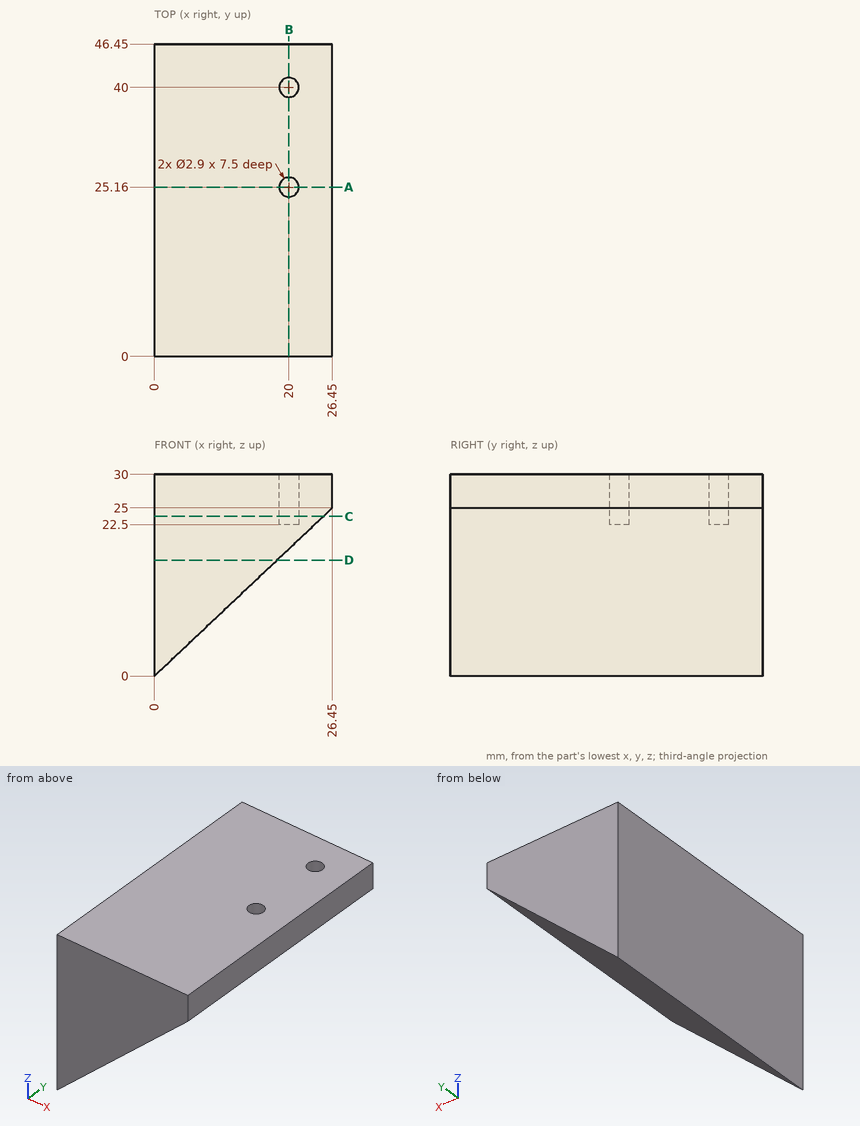
Answer from the drawing. Dimensions are ordinates in mm from the lowest x, y and z of the part. Round coordinates to 2 decimals unless told otherwise and drop trailing zeros. Write each loop counter-clockwise with the first axis right and the second up, starting at its lowest first coordinate (ties: lowest second). Pieces come first, ordered by that corner, then holes.
1. The part is cut by section B-B, the plane x = 20. Determine the outline of the cut face in (y, z).
2. Given pin 1 Ø12 at (y, z) = (15, 6.5) entering from +X (3 decimals); pin 2 Ø10 at (x, y) = (23, 11.5) entering from -Z; pin 3 Ø2.5 at (x, y) = (20, 25) entering from +Z, each flat-ended and moving along its own axis, determine where each tip first touches the part or whether it passes through.
3. The part is cut by section A-A, the plane y = 25.16. Determine the outline of the cut face in (x, z).
4. The part is cut by section D-D, the plane z = 17.25. Determine the outline of the cut face in (x, y), then the cut area to 3 significant figures.
5. Straight lines are drawn through the part: L1, parallel to Y at x = 20, z = 26.25; L2, parallel to Z at x = 17, y = 15; L3, parallel to X at y = 4, z = 5.5. For each, find the intervals that lie inside material, in ascending order.
6. The part is cut by section C-C, the plane z = 23.75. Determine the outline of the cut face in (x, y).
Values:
1. outline: (0, 18.9) - (46.45, 18.9) - (46.45, 30) - (41.45, 30) - (41.45, 22.5) - (38.55, 22.5) - (38.55, 30) - (26.61, 30) - (26.61, 22.5) - (23.71, 22.5) - (23.71, 30) - (0, 30) - close
2. pin 1: stops at x = 13.225
2. pin 2: stops at z = 17.01
2. pin 3: stops at z = 22.5
3. outline: (0, 0) - (26.45, 25) - (26.45, 30) - (21.45, 30) - (21.45, 22.5) - (18.55, 22.5) - (18.55, 30) - (0, 30) - close
4. outline: (0, 0) - (18.25, 0) - (18.25, 46.45) - (0, 46.45) - close
4. area: 848 mm2
5. L1: y = 0 to 23.71, 26.61 to 38.55, 41.45 to 46.45
5. L2: z = 16.07 to 30
5. L3: x = 0 to 5.82
6. outline: (0, 0) - (25.13, 0) - (25.13, 46.45) - (0, 46.45) - close; hole circle Ø2.9 at (20, 25.16); hole circle Ø2.9 at (20, 40)
